Check sheet for the modelled part. Datum: model origin and axes. Units: mm. A direction names the side the tool comes from. Round coordinates to 2 decimals unless told otherwise and drop trailing zeros. Loops run counter-clockwise (first coordinate to the right, second up) from the corner with the lowest first, then second, coordinate; pieces in that order, holes last. Notation, with made-up numbers: (-27.5, -24.75) -> (10.5, -24.75) arc R26 cw to (10.5, -1.75) -> close; hole circle Ø6 at (28.5, 29.5). An arc over 180 degrees is marked (long way). Use one line per item in the form item = value. Start each with the question number.
(1) Set-up check for faces 1 (the flat face through (268, 0, -642)), 2 (the flat face through (284, 3.5, -316)): record each of +Z, -Z, +X, -X, +Y, -Y from which the full face is reachable in a straight line by a thin tool's end or side.
(2) Sectioned sample at A-A (y = -5). Record the cut outline in (x, z).
(3) Material ranges on probe 1 along X at (y, z) = (-5.5, -604); probe 2 along Z at (x, y) = (488, 2.5); probe 3 along X at (y, z) = (0.5, -201), recorded low to high. Write a range as [from, to].
(4) Sectioned sample at B-B (z = -396). Record the cut outline in (x, y), and give its area (3 significant figures).
(5) Go/stop test with flat-tipped pins: pin 1 (3 mm diameter, centred on y = 2, z = -329, fed in from +X); pin 2 (5.5 mm diameter, centred on x = 221.5, z = -640.5, fed in from +Y); pin 3 (7 mm diameter, centred on y = -5.5, z = -644.5, fed in from +X). Record where each tip stops, or that it passes through.
(6) Sectioned sample at C-C (z = -504). Record the cut outline in (x, y), and give its area (3 significant figures).
Autodesk Fusion 360 part; units mm, degrees
sketch "Sketch1" plane through (0, 0, 0) normal (0, 1, 0) x (1, 0, 0)
  line L0 (5, 0) -> (5, 633)
  line L1 (571, 0) -> (571, 184)
  line L2 (539, 633) -> (539, 200)
  line L3 (571, 184) -> (540, 184)
  line L4 (539, 200) -> (539, 184)
  line L5 (539, 184) -> (540, 184)
  line L6 (5, 633) -> (5, 651)
  line L7 (539, 633) -> (539, 651)
  line L8 (539, 651) -> (5, 651)
  line L9 (5, 651) -> (5, 623)
  line L10 (539, 651) -> (539, 623)
  line L11 (5, 0) -> (5, -10)
  line L12 (571, 0) -> (571, -10)
  line L13 (571, -10) -> (5, -10)
  line L14 (5, 633) -> (539, 633)
  dimension "d1" = 633
  dimension "d3" = 184
  dimension "d4" = 534
  dimension "d5" = 433
  dimension "d6" = 31
  dimension "d7" = 16
  dimension "d8" = 18
  dimension "d9" = 18
  dimension "d10" = 28
  dimension "d11" = 28
  dimension "d12" = 10
  dimension "d13" = 10
  dimension "d14" = 566
sketch "Sketch2" plane through (0, 0, 0) normal (0, 1, 0) x (1, 0, 0)
  line L0 (539, 633) -> (539, 200)
  line L1 (5, 633) -> (539, 633)
  line L2 (539, 633) -> (540, 184)
  line L3 (571, 184) -> (540, 184)
  line L4 (540, 184) -> (571, 184)
  line L5 (571, 184) -> (571, -10)
  line L6 (571, -10) -> (5, -10)
  line L7 (5, -10) -> (5, 633)
  point P0 (5, 633)
  point P1 (539, 633)
  point P2 (540, 184)
  point P3 (571, 184)
  point P4 (571, -10)
  point P5 (5, -10)
extrude "Extrude1" add sketch "Sketch1" sketch "Sketch2" against normal blind 9 contours L6 L7 L8 L9 L10 L14 of sketch 2
extrude "Extrude2" add sketch "Sketch2" along normal blind 3.5
Checks:
q1.face_1 = -Z, +X, -X, +Y
q1.face_2 = +Z, -Z, +X, -X, +Y
q2.outline = (5, -651) -> (539, -651) -> (539, -633) -> (540, -184) -> (571, -184) -> (571, 10) -> (5, 10) -> close
q3.probe_1 = [5, 539.06]
q3.probe_2 = [-633, 10]
q3.probe_3 = [5, 539.96]
q4.outline = (5, -9) -> (539.53, -9) -> (539.53, 3.5) -> (5, 3.5) -> close
q4.area = 6,680 mm2
q5.pin_1 = 539.68
q5.pin_2 = 0
q5.pin_3 = 539
q6.outline = (5, -9) -> (539.29, -9) -> (539.29, 3.5) -> (5, 3.5) -> close
q6.area = 6,680 mm2
